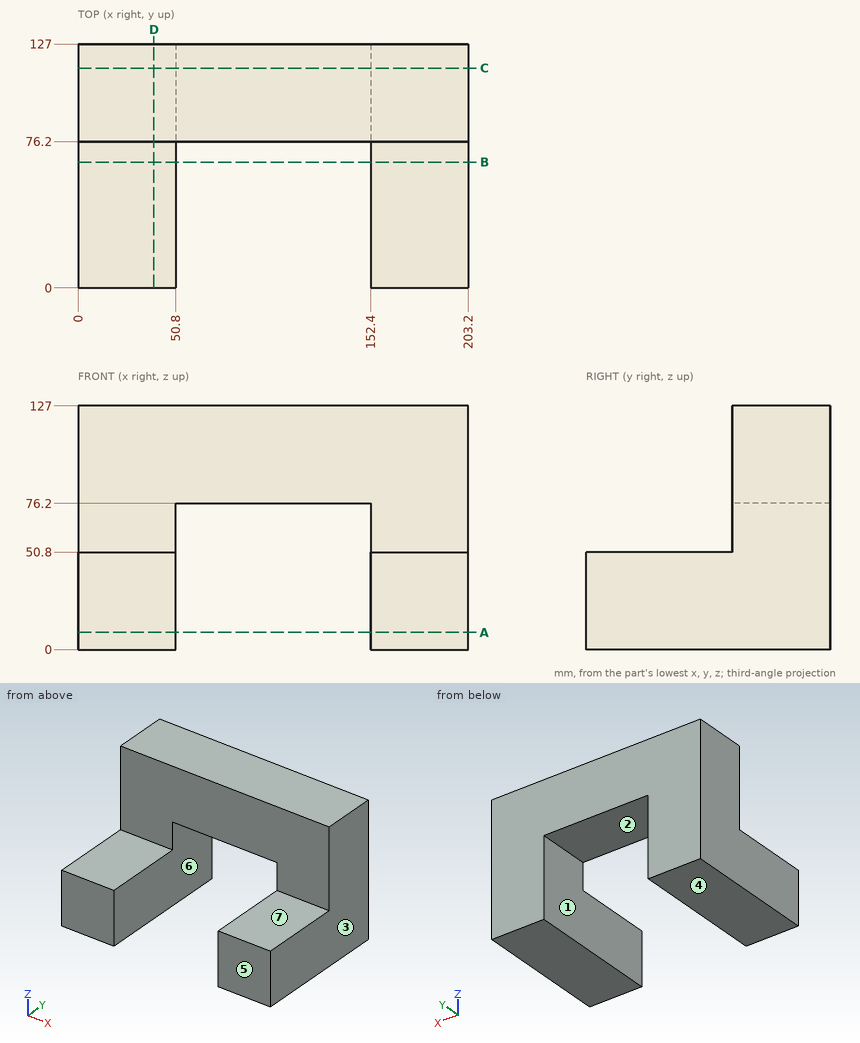
Source: three-view drawing plus pictorial views. Frame: mm from the lowest corner of the part. A direction names the side the tool comes from. Round coordinates to 2 decimals unless told otherwise and drop trailing zeros. Write each loop counter-clockwise with the first axis right and the second up, starting at its lowest first coordinate (ties: lowest second). Pieces come first, ordered by that corner, then holes. Notation, with made-up numbers: M -21,3 L -10,3 A22 ccw -10,20 Z; hole C 33,9 d4. An arc over 180 degrees is marked long. Write each question's results on one line, items separated by ' | '.
Q1. Draft query along X for the marked faces 1, 2, 3 and 4. Return one class per face: released by +X, released by -X, zero draft, split by the parting line, or undercut.
Results:
face 1: undercut | face 2: undercut | face 3: released by +X | face 4: zero draft
Q2. Section query A-A (z = 9). Return loops of the section in (x, y).
Results:
outline: M 0,0 L 50.8,0 L 50.8,127 L 0,127 Z; M 152.4,0 L 203.2,0 L 203.2,127 L 152.4,127 Z
Q3. Section query D-D (x = 39.5). Return loops of the section in (y, z).
Results:
outline: M 0,0 L 127,0 L 127,127 L 76.2,127 L 76.2,50.8 L 0,50.8 Z
Q4. Line query: line 1 along X through (y, z) = (69.5, 31); line 2 along Y through (x, z) = (140.5, 96.5); line 3 along Z through (x, y) = (163, 45.5). Output: solid intervals per line, ascending.
Results:
line 1: x = 0 to 50.8, 152.4 to 203.2 | line 2: y = 76.2 to 127 | line 3: z = 0 to 50.8
Q5. Access query for the marked faces 5, 6 and 7. Directions: +Z, -Z, +X, -X, +Y, -Y. A direction counts if a zero-diameter tool reaches every point of the face in a straight line with its end or side. Return the directions, or none.
Results:
face 5: +Z, -Z, +X, -X, -Y | face 6: -Z, +Y, -Y | face 7: +Z, +X, -X, -Y
Q6. Section query B-B (y = 65.5). Return loops of the section in (x, z).
Results:
outline: M 0,0 L 50.8,0 L 50.8,50.8 L 0,50.8 Z; M 152.4,0 L 203.2,0 L 203.2,50.8 L 152.4,50.8 Z
Q7. Section query C-C (y = 114.5). Return loops of the section in (x, z), and give its area (3 significant figures).
Results:
outline: M 0,0 L 50.8,0 L 50.8,76.2 L 152.4,76.2 L 152.4,0 L 203.2,0 L 203.2,127 L 0,127 Z | area: 18,100 mm^2
Q8. Pin query (flat end, axial travel): P1, Ø23, axis at x = 95.5, z = 101, coming from the -Y side; P2, Ø10, axis at x = 171.5, y = 32, coming from the +Z side. Return the tip coordinate at first contact, or that it passes through.
Results:
P1: stops at y = 76.2 | P2: stops at z = 50.8
